Check sheet for the modelled part. Datum: model origin and axes. Units: mm. Face numbers are marked on the shaded views. A direction names the side the tool comes from. Coordinates: 2 decimals unless noted, no trailing zeros. Loops run counter-clockwise (first coordinate to the right, second up) from the corner with the lowest first, then second, coordinate; pieces in that order, holes last. Notation, with made-up numbers: (81, -8.75) - (94, -8.75) arc R29 ccw to (94, 14.25) - close; hole circle Ø7 at (59, 75). An arc over 180 degrees is marked (long way). Write each question's results on one line, items separated by ' | '. Start each with the question number.
1. Cross-section at D-D (x = 5.25). Record the cut outline in (y, z).
2. Draft check along Z on the marked faces 1, 2, 3 and 4. Enter one of: released by +Z, released by -Z, zero draft, split by the parting line, or undercut.
3. Cross-section at A-A (x = 0). Record the cut outline in (y, z), and give its area (3 significant figures).
4. Cross-section at B-B (y = 11). Record the cut outline in (x, z).
5. Cross-section at C-C (z = 5.5). Record the cut outline in (x, y), and give its area (3 significant figures).
6. Gauge pin test, flat ends, axial feed: P1, Ø8, axis at x = 0, z = 5.5, coming from the -Y side; P2, Ø5.5, axis at x = -1.5, y = 6, coming from the +Z side. Record the tip position at first contact, or that the pin passes through.
7. Tool access check on the marked faces 5, 6 and 7. Record the directions out of +Z, -Z, +X, -X, +Y, -Y that give a thin tool (end or side, any length) a straight path to the whole face; none if there is none.
8. Thickness scan on line 1 (X direction, y = 11.8, z = 5.5); line 2 (Y direction, x = -3.5, z = 9); line 3 (Z direction, x = 0.5, y = 7.25). Record the ranges inside material, lowest first. Write a range as [from, to].
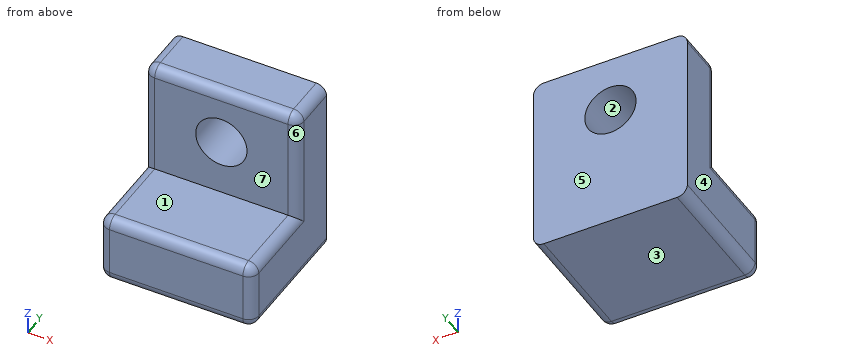
```python
from build123d import *

# Parameters (mm, degrees)
BOSS_EXTRUDE1_DEPTH = 7.5
CUT_EXTRUDE1_REACH  = 20.608
SKETCH2_R           = 2.5
FILLET1_R           = 1


with BuildPart() as part:
    # Sketch1 → Boss-Extrude1 (new, symmetric)
    with BuildSketch(Plane(origin=(0, 0, 0), x_dir=(0, 0, -1), z_dir=(1, 0, 0))):
        Polygon((0, 0), (0, 8), (-11, 8), (-11, 13), (6.7, 13), (6.7, 0), align=None)
    extrude(amount=BOSS_EXTRUDE1_DEPTH, both=True)

    # Sketch2 → Cut-Extrude1 (cut, up to next)
    with BuildSketch(Plane(origin=(0, 13, 0), x_dir=(1, 0, 0), z_dir=(0, 1, 0)), mode=Mode.PRIVATE) as cut_extrude1_sk1:
        with Locations(Location((0, -5.5, 0), (0, 0, 270))):
            Circle(SKETCH2_R)
    cut_extrude1_tool1 = extrude(cut_extrude1_sk1.sketch, amount=-CUT_EXTRUDE1_REACH, mode=Mode.PRIVATE) & part.part
    add(cut_extrude1_tool1.solids().sort_by_distance((0, 13, 5.5))[0], mode=Mode.SUBTRACT)

    # Fillet1
    fillet1_edges = [part.edges().sort_by_distance(p)[0] for p in [
        (0, 0, 0),
        (0, 8, 11),
        (0, 0, -6.7),
        (7.5, 10.5, 11),
        (7.5, 8, 5.5),
        (7.5, 4, 0),
        (7.5, 0, -3.35),
        (-7.5, 4, 0),
        (-7.5, 8, 5.5),
        (-7.5, 10.5, 11),
        (-7.5, 6.5, -6.7),
        (-7.5, 0, -3.35),
        (7.5, 6.5, -6.7),
    ]]
    fillet(fillet1_edges, radius=FILLET1_R)


solid = part.part
```
Established:
1) outline: (0, -5.7) arc R1 ccw to (1, -6.7) - (13, -6.7) - (13, 11) - (9, 11) arc R1 ccw to (8, 10) - (8, 0) - (1, 0) arc R1 ccw to (0, -1) - close
2) face 1: released by +Z | face 2: undercut | face 3: released by -Z | face 4: zero draft
3) outline: (0, -5.7) arc R1 ccw to (1, -6.7) - (13, -6.7) - (13, 3) - (8, 3) - (8, 0) - (1, 0) arc R1 ccw to (0, -1) - close; (8, 8) - (13, 8) - (13, 11) - (9, 11) arc R1 ccw to (8, 10) - close | area: 116 mm^2
4) outline: (-7.5, -5.7) arc R1 ccw to (-6.5, -6.7) - (6.5, -6.7) arc R1 ccw to (7.5, -5.7) - (7.5, 10) arc R1 ccw to (6.5, 11) - (-6.5, 11) arc R1 ccw to (-7.5, 10) - close; hole circle Ø5 at (0, 5.5)
5) outline: (-7.5, 9) arc R1 ccw to (-6.5, 8) - (-2.5, 8) - (-2.5, 13) - (-7.5, 13) - close; (2.5, 8) - (6.5, 8) arc R1 ccw to (7.5, 9) - (7.5, 13) - (2.5, 13) - close | area: 49.6 mm^2
6) P1: y = 8 | P2: z = 10.97
7) face 5: +Z, -Z, +X, -X, +Y | face 6: +Z, +X, -Y | face 7: +Z, +X, -X, -Y
8) line 1: [-7.5, -2.5], [2.5, 7.5] | line 2: [8, 13] | line 3: [-6.7, 0]
